For this review, take the finished solid that the model builds, in its own axes (mm). Give positions to 0.01 mm unless a question says otherwise; leave off trailing zeros. Write each loop counter-clockwise with the first axis right and the second up, starting at its lowest first coordinate (ties: lowest second). Pieces come first, ordered by that corner, then holes. Notation, with made-up numbers: M 26,74 L 81,74 A14 ccw 81,87 Z; hole C 89,-28 d10. An arc over 180 degrees is marked long. Use one line per item in the form item = value. Start each with the question number.
Q1. Consider section C-C on z = 51.5. Write out the cut boundary in (x, y), and give its area (3 significant figures).
Q2. Consider section A-A on x = -75.5. Write out the cut boundary in (y, z), and give its area (3 significant figures).
Q3. Consider section B-B on z = 9.5. Write out the cut boundary in (x, y), and give its area (3 significant figures).
Q4. Clearance check with a flat-ended pin moving along its axis: pin 1 Ø1.9 at (x, y) = (-25.5, 2.5) entering from -Z. State where the tip first meets the part, or that it passes through.
Q5. For probe 1 along X at (y, z) = (5.5, 16); probe 2 along Z at (x, y) = (24.5, 2.75); probe 3 along X at (y, z) = (5.5, 32), list the stretches that pass through material, from the lowest coordinate up. Write a range as [from, to].
Q6. Consider section D-D on x = 57.5. Give the number of separate pieces and of enclosed holes in the cut face, and give its area (3 significant figures).
```python
from build123d import *

# Parameters (mm, degrees)
BOSS_EXTRUDE1_DEPTH = 6.35


with BuildPart() as part:
    # Sketch1 → Boss-Extrude1 (new body)
    with BuildSketch(Plane(origin=(0, 0, 0), x_dir=(1, 0, 0), z_dir=(0, 1, 0))):
        with BuildLine():
            Line((-105, -64.215517859), (-95, -64.215517859))
            Line((-95, -64.215517859), (-95, 12.784482141))
            Line((-95, 12.784482141), (-28, 12.784482141))
            Line((-28, 12.784482141), (-28, -2.215517859))
            Line((-28, -2.215517859), (-19, -2.215517859))
            Line((-19, -2.215517859), (-19, -17.215517859))
            Line((-19, -17.215517859), (46.5, -17.215517859))
            Line((46.5, -17.215517859), (46.5, -0.215517859))
            Line((46.5, -0.215517859), (74.5, -0.215517859))
            Line((74.5, -0.215517859), (74.5, 2.284482141))
            Line((74.5, 2.284482141), (75.995811983, 2.513471084))
            add(Edge.make_bspline(
                [(75.995811983, 2.513471084), (80.478945809, 3.91902752), (86.955874182, 7.104080495), (94.127927524, 13.158287334), (98.453325684, 18.591579482), (101.313529062, 24.942550659), (102.069690209, 32.110869763), (100.125264278, 39.491428955), (95.470460142, 46.405997638), (88.214059069, 52.733240312), (78.176732194, 58.54884887), (65.04289901, 63.866927528), (48.466875468, 68.636346268), (31.498822927, 72.078754421), (18.408481383, 74.071157306), (12.810694193, 74.812442252), (11.34053229, 75)],
                knots=[0, 0, 0, 0, 0.125, 0.1875, 0.25, 0.3125, 0.375, 0.4375, 0.5, 0.5625, 0.625, 0.6875, 0.75, 0.8125, 0.84375, 0.854655416, 0.854655416, 0.854655416, 0.854655416], degree=3))
            Line((11.34053229, 75), (125, 75))
            Line((125, 75), (125, -75))
            Line((125, -75), (-125, -75))
            Line((-125, -75), (-125, 75))
            Line((-125, 75), (-60, 75))
            add(Edge.make_bspline(
                [(74.5, 7.284482141), (106.249859102, 17.238728555), (132.436668925, 69.90318377), (-60, 75)],
                knots=[0, 0, 0, 0, 1, 1, 1, 1], degree=3))
            Line((74.5, 7.284482141), (74.5, 9.784482141))
            Line((74.5, 9.784482141), (46.5, 9.784482141))
            Line((46.5, 9.784482141), (46.5, 48.284482141))
            Line((46.5, 48.284482141), (-19, 48.284482141))
            Line((-19, 48.284482141), (-19, 33.784482141))
            Line((-19, 33.784482141), (-70, 33.784482141))
            Line((-70, 33.784482141), (-70, 23.784482141))
            Line((-70, 23.784482141), (-105, 23.784482141))
            Line((-105, 23.784482141), (-105, -64.215517859))
        make_face()
    extrude(amount=BOSS_EXTRUDE1_DEPTH)


solid = part.part
```
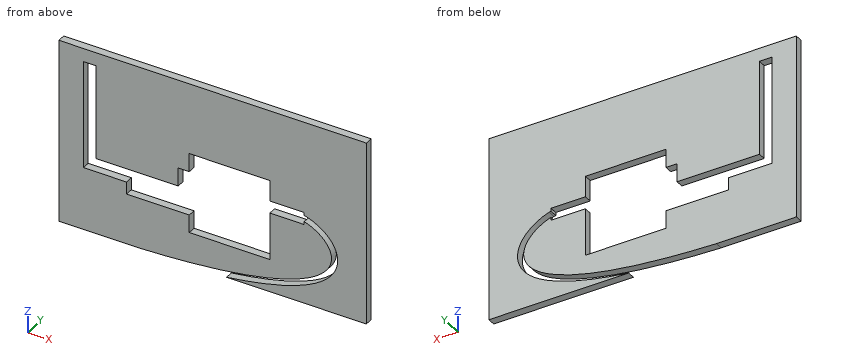
Working result:
q1.outline = M -125,0 L -105,0 L -105,6.35 L -125,6.35 Z; M -95,0 L 125,0 L 125,6.35 L -95,6.35 Z
q1.area = 1,520 mm²
q2.outline = M 0,-75 L 6.35,-75 L 6.35,-23.78 L 0,-23.78 Z; M 0,-12.78 L 6.35,-12.78 L 6.35,75 L 0,75 Z
q2.area = 883 mm²
q3.outline = M -125,0 L -105,0 L -105,6.35 L -125,6.35 Z; M -95,0 L -19,0 L -19,6.35 L -95,6.35 Z; M 46.5,0 L 125,0 L 125,6.35 L 46.5,6.35 Z
q3.area = 1,110 mm²
q4.pin_1 = -73.51
q5.probe_1 = [-125, -105], [-95, -19], [46.5, 125]
q5.probe_2 = [-75, -73.12], [-68.06, -48.28], [17.22, 75]
q5.probe_3 = [-125, -105], [-95, 125]
q6.separate_pieces = 3
q6.enclosed_holes = 0
q6.area = 856 mm²
